Verification items for the finished model (mm, model axes). Coordinates: 2 decimals unless noted, no trailing zeros. Order: outer loops, then holes, each group sorted by start corner. A loop starts at its lowest first (then second) coordinate and runs counter-clockwise, first axis right, second up. Notation, with made-up numbers: M 81,7 L 138,7 A28 cw 138,45 Z; hole C 60.5,74 d4. An arc over 180 degrees is marked long. Answer as a JSON object with one key per item and string values. Group by question number.
(1) Gauge pin test, flat ends, axial feed: pin 1 Ø3 at (x, y) = (-53.5, 39) entering from +Z; pin 2 Ø1.5 at (y, z) = (3, 19.5) entering from +X; pin 3 Ø5 at (x, y) = (-20.5, 3) entering from -Z. Record the tip position at first contact, or that the pin passes through.
(2) Cross-section at B-B (z = 20). Enter the section's corners in (x, y), plus the area to 3 significant figures.
(3) Cross-section at A-A (z = 26). Enter the section's corners in (x, y).
(4) Material ranges on line 1 (X direction, y = 23.5, z = 15); line 2 (X direction, y = 37.5, z = 2); line 3 (Y direction, x = -10.5, z = 19.5), recorded low to high.
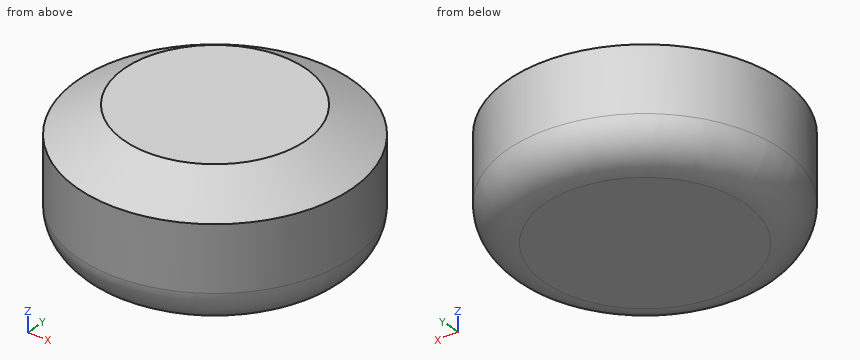
from build123d import *

# Parameters (mm, degrees)
SKETCH_1_R      = 29.65
EXTRUDE_1_DEPTH = 28
CHAMFER_1_SIZE  = 6
CHAMFER_1_SIZE2 = 9.985676894
FILLET_1_R      = 8


with BuildPart() as part:
    # 草图1 → 凸台-拉伸1 (new body)
    with BuildSketch(Plane.XY):
        with Locations((-35.577730584, 22.622481005)):
            Circle(SKETCH_1_R)
    extrude(amount=EXTRUDE_1_DEPTH)

    # 倒角1
    chamfer_1_edges = [part.edges().sort_by_distance(p)[0] for p in [
        (-65.227730584, 22.622481005, 28),
    ]]
    chamfer_1_side = [part.faces().sort_by_distance(p)[0] for p in [
        (-65.227730584, 22.622481005, 14),
    ]]
    chamfer(chamfer_1_edges, length=CHAMFER_1_SIZE, length2=CHAMFER_1_SIZE2, reference=chamfer_1_side[0])

    # 圆角1
    fillet_1_edges = [part.edges().sort_by_distance(p)[0] for p in [
        (-65.227730584, 22.622481005, 0),
    ]]
    fillet(fillet_1_edges, radius=FILLET_1_R)


solid = part.part
Taken from the geometry:
{
 "1": {"pin 1": "stops at z = 26.13", "pin 2": "stops at x = -12.71", "pin 3": "stops at z = 0.02"},
 "2": {"outline": "C -35.58,22.62 d59.3", "area": "2,760 mm²"},
 "3": {"outline": "C -35.58,22.62 d45.99"},
 "4": {"line 1": "x = -65.21 to -5.94", "line 2": "x = -58.04 to -13.12", "line 3": "y = 6.8 to 38.44"}
}
